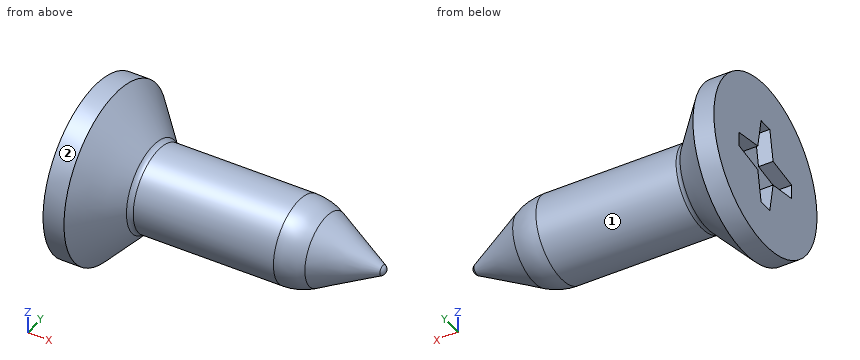
from build123d import *

# Parameters (mm, degrees)
CUT_EXTRUDE1_DEPTH = 0.5


with BuildPart() as part:
    # Sketch1 → Revolve1 (revolve)
    with BuildSketch(Plane.XY):
        with BuildLine():
            Line((0, 0), (0, 2.95))
            Line((0, 2.95), (0.72, 2.95))
            Line((0.72, 2.95), (2.015389317, 1.531420951))
            ThreePointArc((2.015389317, 1.531420951), (2.099115814, 1.47125914), (2.2, 1.45))
            Line((2.2, 1.45), (7.016541593, 1.45))
            ThreePointArc((7.016541593, 1.45), (7.500560514, 1.390547779), (7.955803436, 1.215725683))
            Line((7.955803436, 1.215725683), (9.909315501, 0.176572568))
            ThreePointArc((9.909315501, 0.176572568), (9.986832072, 0.102992143), (10.015389317, 0))
            Line((10.015389317, 0), (0, 0))
        make_face()
    revolve(axis=Axis((-3.974685283, 0, 0), (1, 0, 0)))

    # Sketch2 → Cut-Extrude1 (cut)
    with BuildSketch(Plane.ZY):
        Polygon((-0.25, 1.5), (0.25, 1.5), (0.437370289, 0.437370289), (1.5, 0.25), (1.5, -0.25), (0.437370289, -0.437370289), (0.25, -1.5), (-0.25, -1.5), (-0.437370289, -0.437370289), (-1.5, -0.25), (-1.5, 0.25), (-0.437370289, 0.437370289), align=None)
    extrude(amount=-CUT_EXTRUDE1_DEPTH, mode=Mode.SUBTRACT)


solid = part.part
The model under review builds one solid part; all positions refer to its coordinate system, in mm. Face numbers are marked on the shaded views. A direction names the side the tool comes from. Round coordinates to 2 decimals unless told otherwise and drop trailing zeros. Loops run counter-clockwise (first coordinate to the right, second up) from the corner with the lowest first, then second, coordinate; pieces in that order, holes last. Notation, with made-up numbers: (-34.75, 6.5) -> (6.25, 6.5) arc R18 cw to (6.25, 30.5) -> close; hole circle Ø7 at (-22.5, -15). An arc over 180 degrees is marked (long way). One line per question, with ' | ' between items. Start each with the question number.
Item 1: Machinability: for the marked faces 1 and 2, which of the approach directions +Z, -Z, +X, -X, +Y, -Y give a long, thin tool a straight path to every point of the face, cutting with its end or side? Answer none if there is none.
Item 2: Add section A-A, the plane x = 5.5. Write out the cut boundary in (y, z), then the cut area to 3 significant figures.
Item 3: Add section B-B, the plane x = 8.5. Write out the cut boundary in (y, z), then the cut area to 3 significant figures.
Item 4: For pin 1 (2.5 mm diameter, centred on y = 0.5, z = 0.5, fed in from -X); pin 2 (3 mm diameter, centred on x = 8.5, y = -0.5, fed in from -Z); pin 3 (2 mm diameter, centred on x = 8, y = -0.5, fed in from +Z); pin 4 (1 mm diameter, centred on x = 4.5, z = 1, fed in from -Y), all flat-tipped, find the tip position at first contact; note any pin that passes through.
Item 5: Wall thickness on line 1 along Y through (x, z) = (3.75, 0.8); line 2 along X through (y, z) = (1.15, 1.25); line 3 along X through (y, z) = (-2, -1.8): over which ranges is each line inside the solid? List them lowest first. Write a range as [from, to].
Return value:
1) face 1: +X | face 2: +X, -X
2) outline: circle Ø2.9 at (0, 0) | area: 6.61 mm2
3) outline: circle Ø1.85 at (0, 0) | area: 2.70 mm2
4) pin 1: stops at x = 0 | pin 2: stops at z = -1.45 | pin 3: stops at z = 1.45 | pin 4: stops at y = -1.36
5) line 1: y = [-1.21, 1.21] | line 2: x = [0, 1.86] | line 3: x = [0, 0.96]
